```python
from build123d import *

# Parameters (mm, degrees)
SKETCH1_W               = 26
SKETCH1_H               = 47
SKETCH1_R               = 1.1
BOSS_EXTRUDE1_DEPTH     = 12
SKETCH2_3_W             = 16
SKETCH2_3_H             = 4
BOSS_EXTRUDE2_DEPTH     = 23.5
CUT_EXTRUDE3_DEPTH      = 5
CUT_EXTRUDE3_DEPTH_BACK = 13


with BuildPart() as part:
    # Sketch1 → Boss-Extrude1 (new body)
    with BuildSketch(Plane(origin=(0, 0, 0), x_dir=(1, 0, 0), z_dir=(0, 1, 0))):
        Polygon((-13, -16.375644347), (-13, 23.5), (-20, 23.5), (-20, -14.5), align=None)
        Rectangle(SKETCH1_W, SKETCH1_H)
        with Locations((9, -20)):
            Circle(SKETCH1_R, mode=Mode.SUBTRACT)
        with Locations((-9, -20)):
            Circle(SKETCH1_R, mode=Mode.SUBTRACT)
        with Locations((9, 20)):
            Circle(SKETCH1_R, mode=Mode.SUBTRACT)
        with Locations((-9, 20)):
            Circle(SKETCH1_R, mode=Mode.SUBTRACT)
        Polygon((20, 23.5), (13, 23.5), (13, -16.375644347), (20, -14.5), align=None)
    extrude(amount=-BOSS_EXTRUDE1_DEPTH)

    # Sketch2<3> → Boss-Extrude2 (add)
    with BuildSketch(Plane.XY):
        with Locations((0, 2)):
            Rectangle(SKETCH2_3_W, SKETCH2_3_H)
    extrude(amount=-BOSS_EXTRUDE2_DEPTH)

    # Sketch3 → Cut-Extrude3 (cut, two sides)
    with BuildSketch(Plane(origin=(0, 0, 0), x_dir=(1, 0, 0), z_dir=(0, 1, 0))) as cut_extrude3_sk:
        with BuildLine():
            ThreePointArc((6.1, 14.237262895), (0, 16.25), (-6.1, 14.237262895))
            Line((-6.1, 14.237262895), (-6.1, -2.237262895))
            ThreePointArc((-6.1, -2.237262895), (0, -4.25), (6.1, -2.237262895))
            Line((6.1, -2.237262895), (6.1, 14.237262895))
        make_face()
    extrude(amount=CUT_EXTRUDE3_DEPTH, mode=Mode.SUBTRACT)
    extrude(cut_extrude3_sk.sketch, amount=-CUT_EXTRUDE3_DEPTH_BACK, mode=Mode.SUBTRACT)


solid = part.part
```
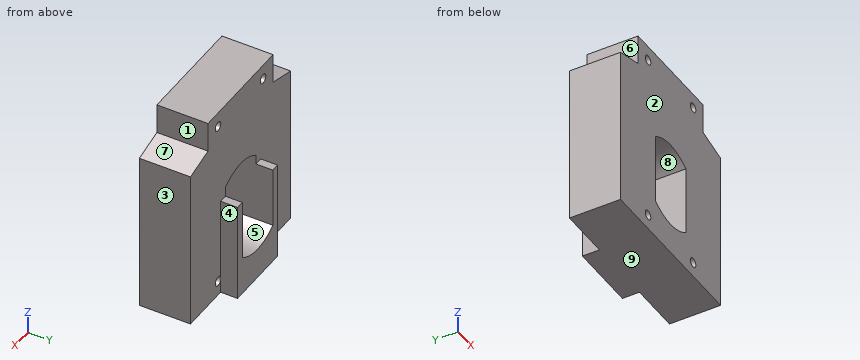
Verification items for the finished model (mm, model axes). Face numbers are marked on the shaded views. A direction names the side the tool comes from. Coordinates: 2 decimals unless noted, no trailing zeros. Loops run counter-clockwise (first coordinate to the right, second up) from the corner with the lowest first, then second, coordinate; pieces in that order, holes last. Notation, with made-up numbers: (-9, -33) - (2, -33) arc R34 cw to (2, 6) - close; hole circle Ø4 at (75.25, 76). An arc over 180 degrees is marked (long way). Answer as a JSON object with one key per item and string values.
(1) Access from +Z, -Z, +X, -X, +Y, -Y to the whole of each face (thin tool, end or side, straight path). Record for the marked faces 1, 2, 3, 4 and 5.
Response:
{"face 1": "+Z, +X, +Y, -Y", "face 2": "+Z, -Z, +X, -X, -Y", "face 3": "+Z, -Z, +X, +Y, -Y", "face 4": "+Z, -Z, +X, +Y", "face 5": "+Y, -Y"}
(2) Cross-section at A-A, the plane z = 20. Record the boundary of the cut face in (x, y), then the cut area to 3 significant figures.
Response:
{"outline": "(-13, -12) - (-10.1, -12) - (-10.1, 0) - (-13, 0) - close; (-7.9, -12) - (7.9, -12) - (7.9, 0) - (-7.9, 0) - close; (10.1, -12) - (13, -12) - (13, 0) - (10.1, 0) - close", "area": "259 mm²"}
(3) Go/stop test with flat-tipped pins: pin 1 Ø2 at (y, z) = (3, -17.5) entering from +X; pin 2 Ø1.5 at (x, y) = (7, 2.5) entering from +Z; pin 3 Ø12 at (x, z) = (2, -5.5) entering from -Y; pin 4 Ø8 at (y, z) = (-9, 21) entering from -X. Record where each tip stops, or that it passes through.
Response:
{"pin 1": "stops at x = 8", "pin 2": "stops at z = 0", "pin 3": "stops at y = -12", "pin 4": "stops at x = -13"}
(4) Mould release check, pull along Z, two halves, no side actions. Record for the marked faces 6, 7, 8 and 9: pulls with the +Z half, pulls with the -Z half, needs draft (parallel to the pull), parting line crosses it, or undercut.
Response:
{"face 6": "needs draft", "face 7": "pulls with the +Z half", "face 8": "undercut", "face 9": "pulls with the -Z half"}
(5) Cross-section at B-B, the plane x = -9. Record the boundary of the cut face in (y, z), then the cut area to 3 significant figures.
Response:
{"outline": "(-12, -23.5) - (0, -23.5) - (0, -21.1) - (-12, -21.1) - close; (-12, -18.9) - (0, -18.9) - (0, 18.9) - (-12, 18.9) - close; (-12, 21.1) - (0, 21.1) - (0, 23.5) - (-12, 23.5) - close", "area": "511 mm²"}
(6) Cross-section at C-C, the plane z = 1.5. Record the boundary of the cut face in (x, y), then the cut area to 3 significant figures.
Response:
{"outline": "(-20, -12) - (-6.1, -12) - (-6.1, 0) - (-20, 0) - close; (6.1, -12) - (20, -12) - (20, 0) - (6.1, 0) - close", "area": "334 mm²"}
(7) Scan lines: line 1 along X through (y, z) = (-2.75, -20); line 2 along Z through (x, y) = (9, -3.25); line 3 along X through (y, z) = (-6, 20). Record each from-to range of solid material in increasing order.
Response:
{"line 1": "x = -20 to -10.1, -7.9 to 7.9, 10.1 to 20", "line 2": "z = -23.5 to -21.1, -18.9 to 18.9, 21.1 to 23.5", "line 3": "x = -13 to -10.1, -7.9 to 7.9, 10.1 to 13"}
(8) Cross-section at D-D, the plane y = -9. Record the boundary of the cut face in (x, z).
Response:
{"outline": "(-20, -23.5) - (20, -23.5) - (20, 14.5) - (13, 16.38) - (13, 23.5) - (-13, 23.5) - (-13, 16.38) - (-20, 14.5) - close; hole circle Ø2.2 at (-9, -20); hole circle Ø2.2 at (-9, 20); hole (-6.1, -14.24) arc R10.25 ccw to (6.1, -14.24) - (6.1, 2.24) arc R10.25 ccw to (-6.1, 2.24) - close; hole circle Ø2.2 at (9, -20); hole circle Ø2.2 at (9, 20)"}
